For this review, use the dimensioned drawing (mm, ordinates from the lowest corner) and the shaded views. A direction names the side the tool comes from. Coordinates: 2 decimals unless noted, no trailing zeros. Order: outer loops, then holes, each group sorted by start corner. A loop starts at its lowest first (then second) coordinate and runs counter-clockwise, first axis right, second up. Notation, with made-up numbers: M 9,67.25 L 36,67.25 A27 cw 36,94.25 Z; hole C 2.5,73 d11. An arc over 180 degrees is marked long. Answer in a Markdown table with one row per item.
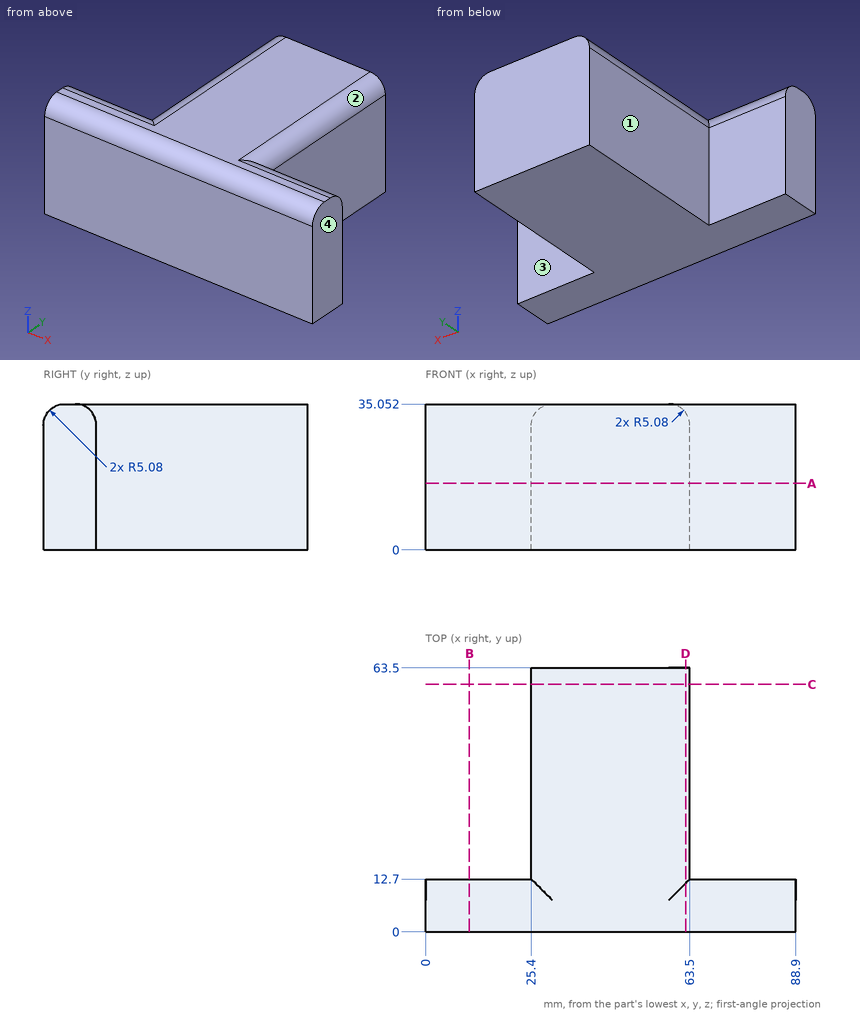
(1) Insertion check: P1, Ø12, axis at x = 57.5, y = 15, coming from the -Z side; P2, Ø1, axis at y = 34, z = 30, coming from the -X side; P3, Ø1.5, axis at x = 67, z = 13, coming from the +Y side; P4, Ø5, axis at y = 27.5, z = 14.5, coming from the +X side. Each pin has a flat end and moves straight along its axis. Give the tip position at first contact, or say it passes through.
Report:
| item | result |
|---|---|
| P1 | z = 0 |
| P2 | x = 25.4 |
| P3 | y = 12.7 |
| P4 | x = 63.5 |
(2) Take a section at B-B (x = 10.5). Write out the cut boundary in (y, z).
Report:
| item | result |
|---|---|
| outline | M 0,0 L 12.7,0 L 12.7,29.97 A5.08 ccw 7.62,35.05 L 5.08,35.05 A5.08 ccw 0,29.97 Z |
(3) Take a section at A-A (z = 16). Write out the cut boundary in (x, y), then the cut area to 3 significant figures.
Report:
| item | result |
|---|---|
| outline | M 0,0 L 88.9,0 L 88.9,12.7 L 63.5,12.7 L 63.5,63.5 L 25.4,63.5 L 25.4,12.7 L 0,12.7 Z |
| area | 3,060 mm^2 |
(4) Machinability: for the marked faces 1, 2, 3 and 4, which of the approach directions +Z, -Z, +X, -X, +Y, -Y give a long, thin tool a straight path to every point of the face, cutting with its end or side? Answer none if there is none.
Report:
| item | result |
|---|---|
| face 1 | +Z, -Z, -X, +Y |
| face 2 | +Z, +X, +Y |
| face 3 | +Z, -Z, +X, +Y |
| face 4 | +Z, -Z, +X, +Y, -Y |
(5) Take a section at C-C (y = 59.5). Write out the cut boundary in (x, z), then the cut area to 3 significant figures.
Report:
| item | result |
|---|---|
| outline | M 25.4,0 L 63.5,0 L 63.5,29.97 A5.08 ccw 58.42,35.05 L 30.48,35.05 A5.08 ccw 25.4,29.97 Z |
| area | 1,320 mm^2 |
(6) To check wall thickness, follow line 1 (X direction, y = 19.5, z = 15.5); line 2 (Y direction, x = 84.5, z = 5.5); line 3 (Z direction, x = 27, y = 9). State the ranges of each line that lie inside material, in increasing order. Write a range as [from, to].
Report:
| item | result |
|---|---|
| line 1 | [25.4, 63.5] |
| line 2 | [0, 12.7] |
| line 3 | [0, 34.86] |
(7) Take a section at D-D (x = 62.5). Write out the cut boundary in (y, z), then the cut area to 3 significant figures.
Report:
| item | result |
|---|---|
| outline | M 0,0 L 63.5,0 L 63.5,33 L 11.7,33 A5.08 ccw 7.62,35.05 L 5.08,35.05 A5.08 ccw 0,29.97 Z |
| area | 2,110 mm^2 |
